Read the model definition and answer for the solid it produces. Units are mm, in the model's axes. Coordinates: 2 decimals unless noted, no trailing zeros. Answer in a Markdown table with one row per item. Add a question column.
Item 1: Given pin 1 Ø0.9 at (y, z) = (122, 2) entering from +X, flat-ended and moving along its own axis, determine where the tip first touches the part or whether it passes through.
Item 2: Section A-A on x = 120 is taken. Count the separate pieces of the cut face and the enclosed holes in it, then the cut area to 3 significant figures.
Item 3: For a pull along Y with two mould halves and no side action, classify faces 1 (the face through (62, 0, 1)), 2 (the face through (62, 76, 3)), 3 (the face through (41.805, 143.714, 1.521)), 4 (the face through (52.5, 123, 1)) as +Y half, -Y half, draft (parallel to the pull), parting line (faces both ways), or undercut.
Item 4: Straight lines are drawn through the part: line 1 (X direction, y = 120, z = 1.8); line 2 (Y direction, x = 44, z = 0.9); line 3 (X direction, y = 99, z = 1.55). For each, find the intervals that lie inside material, in ascending order. Write a range as from..to.
```python
from build123d import *

# Parameters (mm, degrees)
SKETCH1_W           = 125
SKETCH1_H           = 150
BOSS_EXTRUDE1_DEPTH = 3
SKETCH2_R           = 1.6
CUT_EXTRUDE1_DEPTH  = 4
SKETCH3_R           = 1.5
CUT_EXTRUDE2_DEPTH  = 4
SKETCH4_R           = 1.25
CUT_EXTRUDE3_DEPTH  = 4
SKETCH5_W           = 3
SKETCH5_H           = 10
CUT_EXTRUDE4_DEPTH  = 4
SKETCH6_R           = 1.5
CUT_EXTRUDE5_DEPTH  = 4
CUT_EXTRUDE6_DEPTH  = 4
SKETCH8_R           = 1.5
CUT_EXTRUDE7_DEPTH  = 4.0000001
SKETCH9_R           = 1.5
CUT_EXTRUDE8_DEPTH  = 4.0000001
FILLET3_R           = 10
SKETCH10_W          = 21
SKETCH10_H          = 7
CUT_EXTRUDE9_DEPTH  = 4.0000001


with BuildPart() as part:
    # Sketch1 → Boss-Extrude1 (new body)
    with BuildSketch(Plane.XY):
        with Locations((62.5, 75)):
            Rectangle(SKETCH1_W, SKETCH1_H)
    extrude(amount=BOSS_EXTRUDE1_DEPTH)

    # Sketch2 → Cut-Extrude1 (cut, through all)
    with BuildSketch(Plane(origin=(0, 0, 0), x_dir=(-1, 0, 0), z_dir=(0, 0, -1))):
        with Locations((-120, 114.958148689)):
            Circle(SKETCH2_R)
        with Locations((-106, 114.958148689)):
            Circle(SKETCH2_R)
        with Locations((-106, 98.958148689)):
            Circle(SKETCH2_R)
        with Locations((-120, 98.958148689)):
            Circle(SKETCH2_R)
        with Locations((-19, 114.958148689)):
            Circle(SKETCH2_R)
        with Locations((-5, 114.958148689)):
            Circle(SKETCH2_R)
        with Locations((-5, 98.958148689)):
            Circle(SKETCH2_R)
        with Locations((-19, 98.958148689)):
            Circle(SKETCH2_R)
    extrude(amount=-CUT_EXTRUDE1_DEPTH, mode=Mode.SUBTRACT)

    # Sketch3 → Cut-Extrude2 (cut, through all)
    with BuildSketch(Plane(origin=(0, 0, 0), x_dir=(-1, 0, 0), z_dir=(0, 0, -1))):
        with BuildLine():
            ThreePointArc((-79.5, 81.5), (-82.060660172, 82.560660172), (-81, 80))
            Line((-81, 80), (-81, 81.5))
            Line((-81, 81.5), (-79.5, 81.5))
        make_face()
        with BuildLine():
            Line((-81, 81.5), (-81, 80))
            ThreePointArc((-81, 80), (-79.939339828, 80.439339828), (-79.5, 81.5))
            Line((-79.5, 81.5), (-81, 81.5))
        make_face()
        with Locations((-44, 81.5)):
            Circle(SKETCH3_R)
        with Locations((-81, 44.5)):
            Circle(SKETCH3_R)
        with Locations((-44, 44.5)):
            Circle(SKETCH3_R)
    extrude(amount=-CUT_EXTRUDE2_DEPTH, mode=Mode.SUBTRACT)

    # Sketch4 → Cut-Extrude3 (cut, through all)
    with BuildSketch(Plane(origin=(0, 0, 0), x_dir=(-1, 0, 0), z_dir=(0, 0, -1))):
        with Locations((-70.017473816, 14.43752637)):
            Circle(SKETCH4_R)
        with Locations((-55.017473816, 14.43752637)):
            Circle(SKETCH4_R)
    extrude(amount=-CUT_EXTRUDE3_DEPTH, mode=Mode.SUBTRACT)

    # Sketch5 → Cut-Extrude4 (cut, through all)
    with BuildSketch(Plane(origin=(0, 0, 0), x_dir=(-1, 0, 0), z_dir=(0, 0, -1))):
        with Locations((-54, 123.004295886)):
            Rectangle(SKETCH5_W, SKETCH5_H)
        with Locations((-71, 123.004295886)):
            Rectangle(SKETCH5_W, SKETCH5_H)
    extrude(amount=-CUT_EXTRUDE4_DEPTH, mode=Mode.SUBTRACT)

    # Sketch6 → Cut-Extrude5 (cut, through all)
    with BuildSketch(Plane(origin=(0, 0, 0), x_dir=(-1, 0, 0), z_dir=(0, 0, -1))):
        with Locations((-15.5, 135.678181118)):
            Circle(SKETCH6_R)
        with Locations((-109.5, 135.678181118)):
            Circle(SKETCH6_R)
    extrude(amount=-CUT_EXTRUDE5_DEPTH, mode=Mode.SUBTRACT)

    # Sketch7 → Cut-Extrude6 (cut, through all)
    with BuildSketch(Plane.XY.offset(3)):
        with BuildLine():
            Line((18.83856041, 150), (0, 150))
            Line((0, 150), (0, 121.303805561))
            add(Edge.make_bspline(
                [(0, 121.303805561), (5.130729703, 138.554109372), (8.057120528, 143.174726465), (13.293819899, 147.487302418), (18.83856041, 150)],
                knots=[0, 0, 0, 0, 0, 1, 1, 1, 1, 1], degree=4))
        make_face()
        with BuildLine():
            Line((125, 150), (125, 121.303805561))
            add(Edge.make_bspline(
                [(125, 121.303805561), (119.869270297, 138.554109372), (116.942879472, 143.174726465), (111.706180101, 147.487302418), (106.16143959, 150)],
                knots=[0, 0, 0, 0, 0, 1, 1, 1, 1, 1], degree=4))
            Line((106.16143959, 150), (125, 150))
        make_face()
    extrude(amount=-CUT_EXTRUDE6_DEPTH, mode=Mode.SUBTRACT)

    # Sketch8 → Cut-Extrude7 (cut, through all)
    with BuildSketch(Plane.XY.offset(3)):
        with Locations((14.8, 12)):
            Circle(SKETCH8_R)
        with Locations((110.2, 12)):
            Circle(SKETCH8_R)
        with Locations((14.8, 90)):
            Circle(SKETCH8_R)
        with Locations((110.2, 90)):
            Circle(SKETCH8_R)
    extrude(amount=-CUT_EXTRUDE7_DEPTH, mode=Mode.SUBTRACT)

    # Sketch9 → Cut-Extrude8 (cut, through all)
    with BuildSketch(Plane.XY.offset(3)):
        with Locations((42, 142.227223386)):
            Circle(SKETCH9_R)
        with Locations((83, 142.227223386)):
            Circle(SKETCH9_R)
    extrude(amount=-CUT_EXTRUDE8_DEPTH, mode=Mode.SUBTRACT)

    # Fillet3
    fillet3_edges = [part.edges().sort_by_distance(p)[0] for p in [
        (125, 0, 1.5),
        (0, 0, 1.5),
    ]]
    fillet(fillet3_edges, radius=FILLET3_R)

    # Sketch10 → Cut-Extrude9 (cut, through all)
    with BuildSketch(Plane.XY.offset(3)):
        with Locations((62.5, 98.783094858)):
            Rectangle(SKETCH10_W, SKETCH10_H)
    extrude(amount=-CUT_EXTRUDE9_DEPTH, mode=Mode.SUBTRACT)


solid = part.part
```
Results below:
| question | item | result |
|---|---|---|
| 1 | pin 1 | stops at x = 124.93 |
| 2 | separate pieces | 3 |
| 2 | enclosed holes | 0 |
| 2 | area | 383 mm2 |
| 3 | face 1 | -Y half |
| 3 | face 2 | draft |
| 3 | face 3 | undercut |
| 3 | face 4 | undercut |
| 4 | line 1 | x = 0..52.5, 55.5..69.5, 72.5..125 |
| 4 | line 2 | y = 0..43, 46..80, 83..150 |
| 4 | line 3 | x = 0..3.4, 6.6..17.4, 20.6..52, 73..104.4, 107.6..118.4, 121.6..125 |
